```python
from build123d import *

# Parameters (mm, degrees)
F0_W     = 100
F0_H     = 200
F1_DEPTH = 10
F2_SIZE  = 5.08


# Not quite as in the source:
# - the program builds the solid bodies; features that only make, move or delete a surface that nothing else refers to are left out


with BuildPart() as f1:
    # F0 (on Front) → F1 (new body)
    with BuildSketch(Plane.XZ):
        Rectangle(F0_W, F0_H)
    extrude(amount=F1_DEPTH)

    # F2
    f2_edges = [f1.edges().sort_by_distance(p)[0] for p in [
        (-50, -10, 0),
        (0, -10, 100),
        (0, -10, -100),
        (50, -10, 0),
    ]]
    chamfer(f2_edges, length=F2_SIZE)


solid = f1.part
```
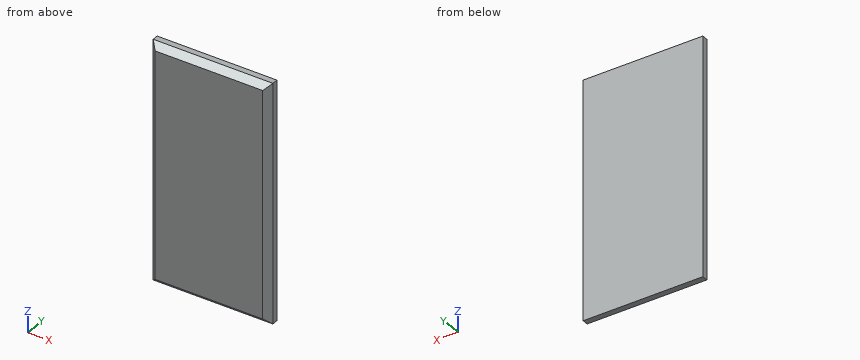
Model file for the job. Use its own axes, mm. Coordinates: 2 decimals unless noted, no trailing zeros. Order: outer loops, then holes, each group sorted by start corner. A loop starts at its lowest first (then second) coordinate and runs counter-clockwise, first axis right, second up. Notation, with made-up numbers: (81, 21.5) - (94, 21.5) arc R14 ccw to (94, 36.5) - close; hole circle Ø10 at (15.5, -32). An arc over 180 degrees is marked (long way). Return JSON: item names as keys, results as strings. Group by question number.
1) Probe line 1 (Z direction, x = 1.5, y = -9.25); line 2 (X direction, y = -6.5, z = 10); line 3 (Z direction, x = 35, y = -7.25). List the from-to ranges inside material, lowest first. Write a range as from..to.
2) Flat gauge pin, fed straight in: P1, Ø1, axis at y = -7.5, z = -40, coming from the +X side. Where does the tip first touch, or does it go through?
3) Saw through at A-A, the plane z = -65. Write the cut outline in (x, y), plus the area to 3 significant figures.
4) Saw through at B-B, the plane y = -7.25. Write the cut outline in (x, z).
Values found:
{
 "1": {"line 1": "z = -95.67..95.67", "line 2": "x = -48.42..48.42", "line 3": "z = -97.67..97.67"},
 "2": {"P1": "stops at x = 47.92"},
 "3": {"outline": "(-50, -4.92) - (-44.92, -10) - (44.92, -10) - (50, -4.92) - (50, 0) - (-50, 0) - close", "area": "974 mm²"},
 "4": {"outline": "(-47.67, -97.67) - (47.67, -97.67) - (47.67, 97.67) - (-47.67, 97.67) - close"}
}
